Design review of the part shown in the three views and the two pictorial views. Dimensions are in mm from the part's minimum x, y and z. A direction names the side the tool comes from. Give positions to 0.01 mm unless a question says otherwise; leave off trailing zeros. Order: outer loops, then holes, each group sorted by start corner. A loop starts at its lowest first (then second) coordinate and runs counter-clockwise, first axis right, second up. Notation, with made-up numbers: M 50.25,64.5 L 79.25,64.5 A14 cw 79.25,85.5 Z; hole C -19.5,16.25 d11. An arc over 180 degrees is marked long. Answer as a JSON object with one key per item and string values.
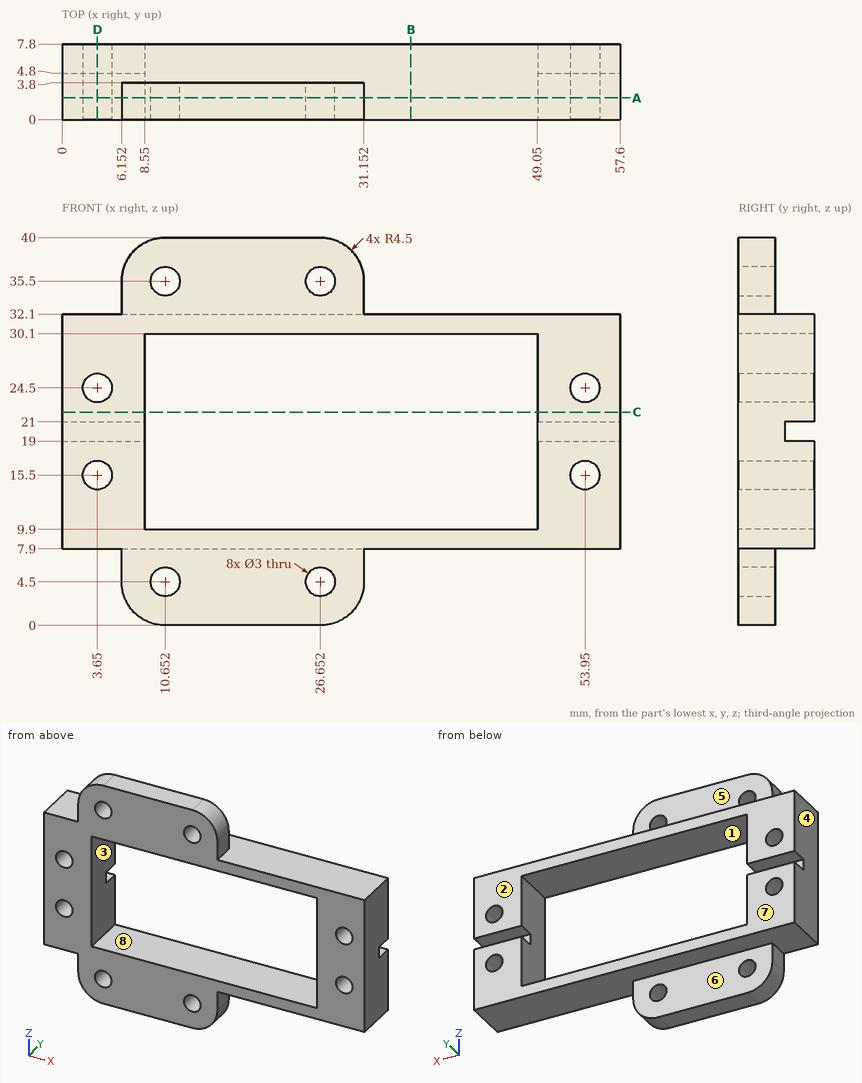
(1) Insertion check: pin 1 (0.9 mm diameter, centred on x = 51.5, y = 6.5, fed in from +Z); pin 2 (1.5 mm diameter, centred on x = 31.5, y = 6, fed in from -Z); pin 3 (4 mm diameter, centred on x = 29, y = 2, fed in from +Z). Each pin has a flat end and moves straight along its axis. Give the tip position at first contact, or say it passes through.
Checked values:
{"pin 1": "stops at z = 32.1", "pin 2": "stops at z = 7.9", "pin 3": "stops at z = 39.99"}
(2) We need section C-C (z = 22). Write out the cut boundary in (x, y).
Checked values:
{"outline": "M 0,0 L 8.55,0 L 8.55,7.8 L 0,7.8 Z; M 49.05,0 L 57.6,0 L 57.6,7.8 L 49.05,7.8 Z"}
(3) We need section A-A (y = 2.25). Count the separate pieces of the cut face and the enclosed holes in it, plus the area to 3 significant figures.
Checked values:
{"separate pieces": "1", "enclosed holes": "9", "area": "897 mm^2"}
(4) We need section D-D (x = 3.65). Write out the cut boundary in (y, z).
Checked values:
{"outline": "M 0,7.9 L 7.8,7.9 L 7.8,14 L 0,14 Z; M 0,17 L 7.8,17 L 7.8,19 L 4.8,19 L 4.8,21 L 7.8,21 L 7.8,23 L 0,23 Z; M 0,26 L 7.8,26 L 7.8,32.1 L 0,32.1 Z"}
(5) Draft analysis for pull direction X (two halves, no side actions). For the marked faces 1, 2, 3 and 4, state which applies: +X half, -X half, draft (parallel to the pull), parting line (faces both ways), or undercut.
Checked values:
{"face 1": "undercut", "face 2": "draft", "face 3": "undercut", "face 4": "-X half"}
(6) Tool access review of the marked faces 5, 6, 7 and 8: name each direction out of +Z, -Z, +X, -X, +Y, -Y from which nothing blocks a thin tool from reaching the whole face with its end or side.
Checked values:
{"face 5": "+Z, +X, -X, +Y", "face 6": "-Z, +X, -X, +Y", "face 7": "+Z, -Z, +X, -X, +Y", "face 8": "+Y, -Y"}
(7) We need section B-B (x = 36). Write out the cut boundary in (y, z).
Checked values:
{"outline": "M 0,7.9 L 7.8,7.9 L 7.8,9.9 L 0,9.9 Z; M 0,30.1 L 7.8,30.1 L 7.8,32.1 L 0,32.1 Z"}
(8) To check wall thickness, follow L1, parallel to Z at x = 54, y = 6.5; L2, parallel to X at y = 1.1, z = 4.5; L3, parallel to X at y = 1, z = 26.5. State the ranges of each line that lie inside material, in increasing order. Write a range as from..to.
Checked values:
{"L1": "z = 7.9..14, 17..19, 21..23, 26..32.1", "L2": "x = 6.15..9.15, 12.15..25.15, 28.15..31.15", "L3": "x = 0..8.55, 49.05..57.6"}
